Here's how the part is built. I have some questions about the finished solid (model axes, mm). A direction names the side the tool comes from. Coordinates: 2 decimals unless noted, no trailing zeros. Write each loop counter-clockwise with the first axis right and the second up, starting at its lowest first coordinate (ties: lowest second). Pieces come first, ordered by that corner, then holes.
Item 1: If we section it at D-D (x = 9): Please give me the cut outline in (y, z).
Item 2: If we section it at C-C (y = 3): Please give me the cut outline in (x, z).
Item 3: If I drill on line 1 (Z direction, x = -3.5, y = 5.25); line 2 (Z direction, x = 13, y = 8.75); line 3 (X direction, y = 9, z = -9), over which ranges is the centre line in solid material (lowest first)?
Item 4: For faces 4 (the face through (0, 5, -1.5)), 5 (the face through (1.267, 4.931, 21.444)), 6 (the face through (0, 0.002, 21)), which set-ups out of +Z, -Z, +X, -X, +Y, -Y let a thin tool reach every point of the face, with its end or its side?
Item 5: We'd pull the mould along X, two halves only. Please class faces 1 (the face through (1.5, 5, 0)), 2 (the face through (0, 0, 4)), 3 (the face through (-1.233, 5.071, 21.444)): +X half, -X half, draft (parallel to the pull), parting line (faces both ways), or undercut.
Item 6: If we section it at B-B (y = 6.75): Please give me the cut outline in (x, z).
Item 7: I'm going to push flat-ended pins straight in: pin 1 Ø5 at (x, y) = (7.5, 8.5) entering from -Z; pin 2 Ø2.5 at (y, z) = (3, 0.5) entering from -X; pin 3 Ø3.5 at (y, z) = (6.5, 0) entering from +X. Where does each tip first touch, or does it pass through?
Item 8: If we section it at A-A (z = 0): Please give me the cut outline in (x, y), then the cut area to 3 significant figures.
from build123d import *

# Parameters (mm, degrees)
SKETCH1_R                  = 20
SKETCH1_W                  = 3
SKETCH1_H                  = 3
BOSS_EXTRUDE1_DEPTH        = 10
BOSS_EXTRUDE2_REACH        = 35
BOSS_EXTRUDE2_START_RADIUS = 20
BOSS_EXTRUDE2_END_RADIUS   = 20


with BuildPart() as part:
    # Sketch1 → Boss-Extrude1 (new body)
    with BuildSketch(Plane(origin=(0, 0, 0), x_dir=(1, 0, 0), z_dir=(0, 1, 0))):
        with Locations(Location((0, 0, 0), (0, 0, 270))):
            Circle(SKETCH1_R)
        Rectangle(SKETCH1_W, SKETCH1_H, mode=Mode.SUBTRACT)
    extrude(amount=BOSS_EXTRUDE1_DEPTH)

    # Boss-Extrude2: from a cylinder face, 35 long prism both ways, kept between that surface and its translate by the depth
    boss_extrude2_start = Plane(origin=(0, 3.334512, 0), z_dir=(0, -1, 0)) * Cylinder(BOSS_EXTRUDE2_START_RADIUS, 111, mode=Mode.PRIVATE)
    boss_extrude2_end = Plane(origin=(0, 3.334512, 3), z_dir=(0, -1, 0)) * Cylinder(BOSS_EXTRUDE2_END_RADIUS, 111, mode=Mode.PRIVATE)
    # Sketch2 → Boss-Extrude2 (add, from a surface)
    with BuildSketch(Plane.XY, mode=Mode.PRIVATE) as boss_extrude2_sk1:
        Polygon((0, 10), (-2.5, 0.001767652), (2.5, 0.001767652), align=None)
    boss_extrude2_tool1 = extrude(boss_extrude2_sk1.sketch, amount=BOSS_EXTRUDE2_REACH, both=True, mode=Mode.PRIVATE)
    add(((boss_extrude2_tool1 - boss_extrude2_start) & boss_extrude2_end).solids().sort_by_distance((0, 3.334512, 21.421567))[0])


solid = part.part
Answer list:
1. outline: (0, -17.86) - (10, -17.86) - (10, 17.86) - (0, 17.86) - close
2. outline: (-1.75, 19.92) arc R20 ccw (long way) to (1.75, 19.92) - (1.75, 22.92) arc R20 ccw to (-1.75, 22.92) - close; hole (-1.5, -1.5) - (1.5, -1.5) - (1.5, 1.5) - (-1.5, 1.5) - close
3. line 1: z = -19.69 to 19.69
3. line 2: z = -15.2 to 15.2
3. line 3: x = -17.86 to 17.86
4. face 4: +Y, -Y
4. face 5: +Z, +X, +Y
4. face 6: +Z, -Z, +X, -X, -Y
5. face 1: undercut
5. face 2: draft
5. face 3: -X half
6. outline: (-0.81, 19.98) arc R20 ccw (long way) to (0.81, 19.98) - (0.81, 22.98) arc R20 ccw to (-0.81, 22.98) - close; hole (-1.5, -1.5) - (1.5, -1.5) - (1.5, 1.5) - (-1.5, 1.5) - close
7. pin 1: stops at z = -19.36
7. pin 2: stops at x = -20
7. pin 3: stops at x = 20
8. outline: (-20, 0) - (-1.5, 0) - (-1.5, 10) - (-20, 10) - close; (1.5, 0) - (20, 0) - (20, 10) - (1.5, 10) - close
8. area: 370 mm2
